The drawing under review shows one solid part. Ordinate dimensions are in mm from its lowest x, y, z. Coordinates: 2 decimals unless noted, no trailing zeros. Order: outer loops, then holes, each group sorted by start corner. A loop starts at its lowest first (then second) coordinate and runs counter-clockwise, first axis right, second up. Notation, with made-up numbers: (75, -23) -> (134, -23) arc R9 cw to (134, -10) -> close; hole circle Ø1 at (56, 61.5). An arc over 180 degrees is marked (long way). Write item = value, one per line.
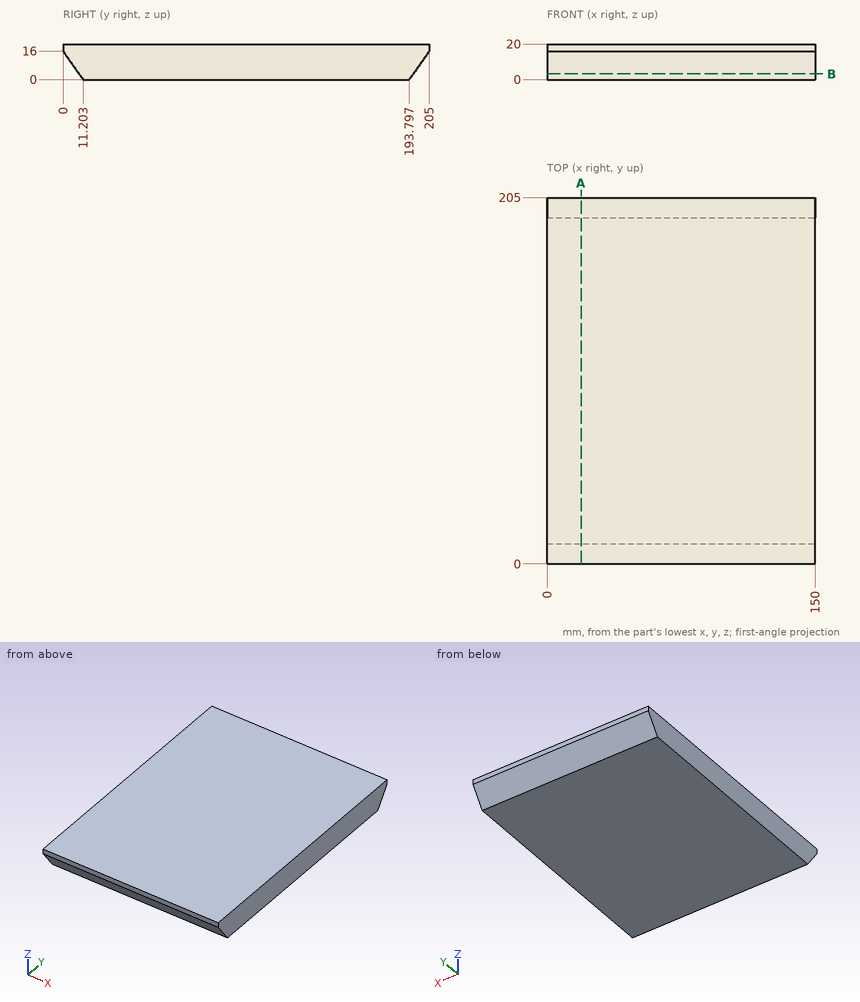
(1) Insertion check: pin 1 (12 mm diameter, centred on x = 130.5, z = 3, fed in from +Y); pin 2 (10 mm diameter, centred on x = 120, z = 7.5, fed in from +Y); pin 3 (12 mm diameter, centred on x = 103, z = 11.5, fed in from +Y). Each pin has a flat end and moves straight along its axis. Give the tip position at first contact, or say it passes through.
Report:
pin_1 = 200.1
pin_2 = 202.55
pin_3 = 205
(2) For L1, parallel to Y at x = 25, z = 10.25 (1 decimal); L2, parallel to Y at x = 102.5, z = 5, list the stretches that pass through material, from the lowest coordinate up.
Report:
L1 = 4 to 201
L2 = 7.7 to 197.3
(3) We need section A-A (x = 19). Write out the cut boundary in (y, z), and give its area (3 significant figures).
Report:
outline = (0, 16) -> (11.2, 0) -> (193.8, 0) -> (205, 16) -> (205, 20) -> (0, 20) -> close
area = 3,920 mm²
(4) We need section B-B (z = 3.25). Write out the cut boundary in (x, y).
Report:
outline = (0, 8.93) -> (150, 8.93) -> (150, 196.07) -> (0, 196.07) -> close
